Autodesk Inventor part; units mm, degrees
ref_plane "YZ Plane" through (0, 0, 0) normal (1, 0, 0) x (0, 1, 0)
ref_plane "XZ Plane" through (0, 0, 0) normal (0, 1, 0) x (-1, 0, 0)
ref_plane "XY Plane" through (0, 0, 0) normal (0, 0, 1) x (1, 0, 0)
sketch "Sketch1" plane through (0, 0, 0) normal (0, 0, 1) x (1, 0, 0)
  line L0 (-177.8, -19.05) -> (177.8, -19.05)
  line L1 (177.8, -19.05) -> (177.8, 19.05)
  line L2 (177.8, 19.05) -> (-177.8, 19.05)
  line L3 (-177.8, 19.05) -> (-177.8, -19.05)
  line L4 (-177.8, -19.05) -> (177.8, 19.05) construction
  line L5 (177.8, -19.05) -> (-177.8, 19.05) construction
  point P0 (0, 0)
  point P1 (0, 0)
  dimension "d31" = 355.6
  dimension "d32" = 38.1
extrude "Plate1" add sketch "Sketch1" along normal blind 6.35
sketch "Sketch3" plane through (177.8, -23.0251, 7.4151) normal (0, -0.5, -0.8660254) x (1, 0, 0)
  line L0 (-355.6, 0) -> (0, 0)
  line L1 (0, 0) -> (0, 125.3998)
  line L2 (0, 125.3998) -> (-355.6, 125.3998)
  line L3 (-355.6, 125.3998) -> (-355.6, 0)
edge flange "Flange2" height 139.7 angle 30 thickness 6.35 bend radius 7.9502 thickness toward (0, -0.5, -0.8660254) relief tear relief width 6.35 relief depth 3.175 edges at (0, -19.05, 6.35) wall of the first edge with corners at (-177.8, -23.0251, 7.4151) (177.8, -23.0251, 7.4151) (177.8, -131.6245, 70.115) (-177.8, -131.6245, 70.115)
bend "Bend2"
corner "Corner2"
fillet "Corner Round1" radius 6.35 2 edges at (177.8, 19.05, 3.175) (-177.8, 19.05, 3.175)
fillet "Corner Round2" radius 38.1 2 edges at (177.8, -133.212, 67.3654) (-177.8, -133.212, 67.3654)
sketch "Sketch4" plane through (-177.8, -23.0251, 7.4151) normal (0, 0.5, 0.8660254) x (1, 0, 0)
  line L0 (152.4, -9.5123) -> (203.2, -9.5123)
  line L1 (215.9, -22.2123) -> (215.9, -85.7123)
  line L2 (203.2, -98.4123) -> (152.4, -98.4123)
  line L3 (139.7, -85.7123) -> (139.7, -22.2123)
  line L4 (139.7, -9.5123) -> (215.9, -98.4123) construction
  line L5 (215.9, -9.5123) -> (139.7, -98.4123) construction
  line L6 (38.1, -125.3998) -> (317.5, -125.3998) construction
  arc A0 (152.4, -9.5123) -> (139.7, -22.2123) centre (152.4, -22.2123) ccw
  arc A1 (215.9, -22.2123) -> (203.2, -9.5123) centre (203.2, -22.2123) ccw
  arc A2 (203.2, -98.4123) -> (215.9, -85.7123) centre (203.2, -85.7123) ccw
  arc A3 (139.7, -85.7123) -> (152.4, -98.4123) centre (152.4, -85.7123) ccw
  line L7 (63.5, -79.3623) -> (63.5, -28.5623) construction
  line L8 (50.8, -79.3623) -> (50.8, -28.5623)
  line L9 (76.2, -28.5623) -> (76.2, -79.3623)
  arc A4 (50.8, -79.3623) -> (76.2, -79.3623) centre (63.5, -79.3623) ccw
  arc A5 (76.2, -28.5623) -> (50.8, -28.5623) centre (63.5, -28.5623) ccw
  line L10 (0, -87.2998) -> (0, 0)
  line L11 (177.8, -53.9623) -> (177.8, -125.3998) construction
  line L12 (292.1, -79.3623) -> (292.1, -28.5623) construction
  line L13 (304.8, -79.3623) -> (304.8, -28.5623)
  line L14 (279.4, -28.5623) -> (279.4, -79.3623)
  arc A6 (279.4, -79.3623) -> (304.8, -79.3623) centre (292.1, -79.3623) ccw
  arc A7 (304.8, -28.5623) -> (279.4, -28.5623) centre (292.1, -28.5623) ccw
  point P0 (63.5, -53.9623)
  dimension "d45" = 26.9875
  dimension "d46" = 76.2
  dimension "d47" = 88.9
  dimension "d50" = 12.7
  dimension "d51" = 12.7
  dimension "d52" = 50.8
  dimension "d53" = 63.5
  dimension "d54" = 25.4
extrude "Cut1" cut sketch "Sketch4" against normal blind 6.35
equation "\"d48\" = Thickness"
equation "\"d15\" = Thickness"
equation "\"d33\" = BendReliefWidth"
equation "\"d34\" = BendReliefDepth"
equation "\"d35\" = MinimumRemnant"
equation "\"d36\" = TransitionRadius"
equation "\"d39\" = BendRadius"
equation "\"d40\" = CornerReliefSize"
equation "\"d41\" = GapSize"
equation "\"d42\" = JacobiRadiusSize"
equation "\"BendReliefWidth\" = Thickness"
equation "\"BendReliefDepth\" = 0.5 * Thickness"
equation "\"CornerReliefSize\" = 4 * Thickness"
equation "\"MinimumRemnant\" = 2 * Thickness"
equation "\"TransitionRadius\" = BendRadius"
equation "\"JacobiRadiusSize\" = Thickness"
equation "\"GapSize\" = Thickness"
properties part number "Model-4_Sheet Stifferner" material "SS304"
Check sheet for the modelled part. Datum: model origin and axes. Units: mm. A direction names the side the tool comes from. Round coordinates to 2 decimals unless told otherwise and drop trailing zeros. Order: outer loops, then holes, each group sorted by start corner. A loop starts at its lowest first (then second) coordinate and runs counter-clockwise, first axis right, second up. Notation, with made-up numbers: (12, 65.25) - (45, 65.25) arc R22 cw to (45, 79.25) - close; hole circle Ø8 at (82.5, 68). An arc over 180 degrees is marked (long way). Answer as CSV lines item,"result". Start each with the question number.
1) Section check D-D (y = -15.5). Record the cut outline in (x, z).
2) Tool access check on faces 1 (the face through (-175.89, 17.24, 3.22)), 2 (the face through (-2, 0, 6.35)), 3 (the face through (34.48, -36.14, 11.37)), 4 (the face through (34.28, -106.68, 52.1)). Record the directions out of +Z, -Z, +X, -X, +Y, -Y that give a thin tool (end or side, any length) a straight path to the whole face; none if there is none.
3) Depth check by flat-ended pin: pin 1 (12 mm diameter, centred on x = -28.5, y = -103.5, fed in from +Z); pin 2 (9.5 mm diameter, centred on y = -65.5, z = 32.5, fed in from +X); pin 3 (1 mm diameter, centred on x = -130, z = 19, fed in from +Y); pin 4 (3 mm diameter, centred on x = -77.5, y = -113.5, fed in from +Z). Enter the tip coordinate at first touch or a pass-through.
4) Scan lines: probe 1 along Z at (x, y) = (48, 1); probe 2 along Z at (x, y) = (-89, -72.5); probe 3 along Y at (x, z) = (157, 40.5). Record each from-to range of solid material in increasing order.
5) Section check C-C (z = 27.5). Record the cut outline in (x, y).
6) Draft check along X on faces 5 (the face through (2.5, -22.8, 0.5)), 6 (the face through (-34.281, -35.965, 11.271)), 7 (the face through (166.935, -123.312, 61.598)). Enter one of: +X half, -X half, draft (parallel to the pull), parting line (faces both ways), or undercut.
Determined:
1,outline,"(-177.8, 0) - (177.8, 0) - (177.8, 6.35) - (-177.8, 6.35) - close"
2,face 1,"+Z, -Z, -X, +Y"
2,face 2,"+Z, +X, -X, +Y"
2,face 3,"+Z, -Y"
2,face 4,"-Z, +Y"
3,pin 1,"z = 57.34"
3,pin 2,"x = 177.8"
3,pin 3,"y = -42.22"
3,pin 4,"z = 60.52"
4,probe 1,"0 to 6.35"
4,probe 2,"28.65 to 35.98"
4,probe 3,"-93.03 to -80.33"
5,outline,"(-177.8, -70.51) - (-127, -70.51) - (-127, -57.81) - (-177.8, -57.81) - close; (-101.6, -70.51) - (-38.1, -70.51) - (-38.1, -57.81) - (-101.6, -57.81) - close; (38.1, -70.51) - (101.6, -70.51) - (101.6, -57.81) - (38.1, -57.81) - close; (127, -70.51) - (177.8, -70.51) - (177.8, -57.81) - (127, -57.81) - close"
6,face 5,"draft"
6,face 6,"undercut"
6,face 7,"+X half"
